```python
from build123d import *

# Parameters (mm, degrees)
BOSS_EXTRUDE1_DEPTH = 3
SKETCH2_R           = 1.75
SKETCH2_R_2         = 12.5
SKETCH2_R_3         = 2.75
CUT_EXTRUDE1_DEPTH  = 3
SKETCH3_R           = 4.75
SKETCH3_R_2         = 2.75
BOSS_EXTRUDE2_DEPTH = 4.5
SKETCH4_R           = 2.25
BOSS_EXTRUDE3_DEPTH = 3
FILLET1_R           = 5
SKETCH5_R           = 2.25
CUT_EXTRUDE2_DEPTH  = 4


with BuildPart() as part:
    # Sketch1 → Boss-Extrude1 (new body)
    with BuildSketch(Plane.XY):
        with BuildLine():
            Line((-65, 25), (65, 25))
            ThreePointArc((65, 25), (68.535533906, 23.535533906), (70, 20))
            Line((70, 20), (70, -20))
            ThreePointArc((70, -20), (68.535533906, -23.535533906), (65, -25))
            Line((65, -25), (-65, -25))
            ThreePointArc((-65, -25), (-68.535533906, -23.535533906), (-70, -20))
            Line((-70, -20), (-70, 20))
            ThreePointArc((-70, 20), (-68.535533906, 23.535533906), (-65, 25))
        make_face()
    extrude(amount=BOSS_EXTRUDE1_DEPTH)

    # Sketch2 → Cut-Extrude1 (cut)
    with BuildSketch(Plane.XY.offset(3)):
        with Locations((-64.75, 15.75)):
            Circle(SKETCH2_R)
        with Locations((-33.25, 15.75)):
            Circle(SKETCH2_R)
        with Locations((-64.75, -15.75)):
            Circle(SKETCH2_R)
        with Locations((-33.25, -15.75)):
            Circle(SKETCH2_R)
        with Locations((-49, 0)):
            Circle(SKETCH2_R_2)
        with Locations((57, 15)):
            Circle(SKETCH2_R_3)
        with Locations((57, -15)):
            Circle(SKETCH2_R_3)
        with Locations((-5, 0)):
            Circle(SKETCH2_R_3)
    extrude(amount=-CUT_EXTRUDE1_DEPTH, mode=Mode.SUBTRACT)

    # Sketch3 → Boss-Extrude2 (add)
    with BuildSketch(Plane.XY.offset(3)):
        with Locations((57, 15)):
            Circle(SKETCH3_R)
        with Locations((57, 15)):
            Circle(SKETCH3_R_2, mode=Mode.SUBTRACT)
        with Locations((-5, 0)):
            Circle(SKETCH3_R)
        with Locations((-5, 0)):
            Circle(SKETCH3_R_2, mode=Mode.SUBTRACT)
        with Locations((57, -15)):
            Circle(SKETCH3_R)
        with Locations((57, -15)):
            Circle(SKETCH3_R_2, mode=Mode.SUBTRACT)
    extrude(amount=BOSS_EXTRUDE2_DEPTH)

    # Sketch4 → Boss-Extrude3 (add)
    with BuildSketch(Plane.XY):
        with BuildLine():
            Line((70, 10), (70, -10))
            Line((70, -10), (80, -10))
            ThreePointArc((80, -10), (90, 0), (80, 10))
            Line((80, 10), (70, 10))
        make_face()
        with Locations((80, 0)):
            Circle(SKETCH4_R, mode=Mode.SUBTRACT)
    extrude(amount=BOSS_EXTRUDE3_DEPTH)

    # Fillet1
    fillet1_edges = [part.edges().sort_by_distance(p)[0] for p in [
        (70, -10, 1.5),
        (70, 10, 1.5),
    ]]
    fillet(fillet1_edges, radius=FILLET1_R)

    # Sketch5 → Cut-Extrude2 (cut, through all)
    with BuildSketch(Plane.XY.offset(3)):
        with Locations((16, 0)):
            Circle(SKETCH5_R)
        with Locations((36, 0)):
            Circle(SKETCH5_R)
    extrude(amount=-CUT_EXTRUDE2_DEPTH, mode=Mode.SUBTRACT)


solid = part.part
```
Input: part model. Units: mm. Frame: model coordinates. A direction names the side the tool comes from. Give positions to 0.01 mm unless a question says otherwise; leave off trailing zeros. Order: outer loops, then holes, each group sorted by start corner. A loop starts at its lowest first (then second) coordinate and runs counter-clockwise, first axis right, second up. Notation, with made-up numbers: M 77.25,10.25 L 83.25,10.25 A16 cw 83.25,27.25 Z; hole C 77,-3 d8. An arc over 180 degrees is marked long. Return JSON: item names as keys, results as strings.
1) Section query B-B on y = 0. Output: boundary loops of the cut face in (x, z).
Taken from the geometry:
{"outline": "M -70,0 L -61.5,0 L -61.5,3 L -70,3 Z; M -36.5,0 L -7.75,0 L -7.75,7.5 L -9.75,7.5 L -9.75,3 L -36.5,3 Z; M -2.25,0 L 13.75,0 L 13.75,3 L -0.25,3 L -0.25,7.5 L -2.25,7.5 Z; M 18.25,0 L 33.75,0 L 33.75,3 L 18.25,3 Z; M 38.25,0 L 77.75,0 L 77.75,3 L 38.25,3 Z; M 82.25,0 L 90,0 L 90,3 L 82.25,3 Z"}
2) Access query for faces 1 (the face through (-6.03, -4.637, 5.219)), 2 (the face through (-63.081, 16.276, 1.521)), 3 (the face through (70, -17, 1)), 4 (the face through (78, 10, 1)). Directions: +Z, -Z, +X, -X, +Y, -Y. A direction counts if a zero-diameter tool reaches every point of the face in a straight line with its end or side. Return the directions, or none.
Taken from the geometry:
{"face 1": "+Z", "face 2": "+Z, -Z", "face 3": "+Z, -Z, +X, -Y", "face 4": "+Z, -Z, +X, +Y"}
3) Line query: L1, parallel to Y at x = -33.25, z = 2.4; L2, parallel to Y at x = 57, z = 4.3; L3, parallel to Y at x = 36, z = 1.05. Output: solid intervals per line, ascending. Write a range as [from, to].
Taken from the geometry:
{"L1": "y = [-25, -17.5], [-14, 14], [17.5, 25]", "L2": "y = [-19.75, -17.75], [-12.25, -10.25], [10.25, 12.25], [17.75, 19.75]", "L3": "y = [-25, -2.25], [2.25, 25]"}
4) Section query C-C on x = -5. Output: boundary loops of the cut face in (y, z), and give its area (4 significant figures).
Taken from the geometry:
{"outline": "M -25,0 L -2.75,0 L -2.75,7.5 L -4.75,7.5 L -4.75,3 L -25,3 Z; M 2.75,0 L 25,0 L 25,3 L 4.75,3 L 4.75,7.5 L 2.75,7.5 Z", "area": "151.5 mm2"}
5) Section query A-A on z = 4.5. Output: boundary loops of the cut face in (x, y), and give its area (3 significant figures).
Taken from the geometry:
{"outline": "C -5,0 d9.5; C 57,-15 d9.5; C 57,15 d9.5; hole C -5,0 d5.5; hole C 57,-15 d5.5; hole C 57,15 d5.5", "area": "141 mm2"}
6) Contact query for flat-ended pins moving along their axis: pin 1 (0.9 mm diameter, centred on y = -18, z = 1, fed in from +X); pin 2 (3.5 mm diameter, centred on x = 76.5, z = 1.5, fed in from +Y); pin 3 (2 mm diameter, centred on x = 67, z = 2, fed in from +Y); pin 4 (3 mm diameter, centred on x = -33.25, y = -15.75, fed in from +Z). Output: stop coordinate, or through.
Taken from the geometry:
{"pin 1": "stops at x = 70", "pin 2": "stops at y = 10.01", "pin 3": "stops at y = 24.9", "pin 4": "passes through"}
7) Mould query, pull axis X, two halves, no side actions, for faces 5 (the face through (-70, 0, 1)), 6 (the face through (71, -12, 2)), 7 (the face through (82.08, -0.86, 1.48)). Classes: released by +X, released by -X, zero draft, split by the parting line, or undercut.
Taken from the geometry:
{"face 5": "released by -X", "face 6": "released by +X", "face 7": "undercut"}
8) Section query D-D on y = 8.5. Output: boundary loops of the cut face in (x, z), and give its area (3 significant figures).
Taken from the geometry:
{"outline": "M -70,0 L -58.17,0 L -58.17,3 L -70,3 Z; M -39.83,0 L 85.27,0 L 85.27,3 L -39.83,3 Z", "area": "411 mm2"}
